from build123d import *

# Parameters (mm, degrees)
SKETCH_R    = 4
PAD_DEPTH   = 14
SKETCH001_R = 2.5
HOLE_DEPTH  = 25
HOLE_TIPS_R = 2.5
FILLET_R    = 1


with BuildPart() as part:
    # Sketch → Pad (new body)
    with BuildSketch(Plane.XY):
        Polygon((0, 0), (25, 0), (25, 8), (14, 8), (14, 36), (0, 36), align=None)
        with Locations((7, 28)):
            Circle(SKETCH_R, mode=Mode.SUBTRACT)
    extrude(amount=PAD_DEPTH)

    # Sketch001 (on Face6 of Pad) → Hole (cut)
    with BuildSketch(Plane(origin=(0, 0, 0), x_dir=(0, -1, 0), z_dir=(-1, 0, 0))):
        with Locations((-13, 7)):
            Circle(SKETCH001_R)
    extrude(amount=-HOLE_DEPTH, mode=Mode.SUBTRACT)

    # Hole tips → Hole tip 1 section 0
    with BuildSketch(Plane(origin=(25, 0, 0), x_dir=(0, -1, 0), z_dir=(-1, 0, 0)), mode=Mode.PRIVATE) as hole_tip_1_s0:
        with Locations((-13, 7)):
            Circle(HOLE_TIPS_R)
    loft([hole_tip_1_s0.sketch, Vertex(26.502152, 13, 7)], mode=Mode.SUBTRACT)

    # Fillet
    fillet_edges = [part.edges().sort_by_distance(p)[0] for p in [
        (14, 8, 7),
        (14, 36, 7),
        (0, 36, 7),
        (25, 8, 7),
    ]]
    fillet(fillet_edges, radius=FILLET_R)


solid = part.part
Can you work these out from the model? Positions are in its coordinate system, mm. A direction names the side the tool comes from. Coordinates: 2 decimals unless noted, no trailing zeros. Order: outer loops, then holes, each group sorted by start corner. A loop starts at its lowest first (then second) coordinate and runs counter-clockwise, first axis right, second up. Notation, with made-up numbers: (55, 77) - (95, 77) arc R26 ccw to (95, 103) - close; hole circle Ø6 at (8, 0). An arc over 180 degrees is marked (long way). Answer as a JSON object with one key per item and string values. Group by question number.
Q1. Imagine slicing it at C-C (x = 11.75). Please give me the cut outline in (y, z), and give its area (3 significant figures).
Q2. Imagine slicing it at A-A (z = 7). Please give me the cut outline in (x, y), and give its area (3 significant figures).
Q3. On a 3-axis mill with a long thin cutter (end or side, diameter ignored), from which of +Z, -Z, +X, -X, +Y, -Y can I reach the whole of each face in a straight line? I mean faces 1 (the face through (0, 18, 7)), 2 (the face through (14, 22, 7)). Say none if no direction works.
Q4. Imagine slicing it at B-B (y = 13). Please give me the cut outline in (x, z).
Q5. I need wall thicknesses on line 1 (Y direction, x = 12, z = 8.5); line 2 (Y direction, x = 4.75, z = 5); line 3 (Z direction, x = 5, y = 13). Which ranges of each line are inside material? Lowest first, please. Write a range as from..to.
Q6. Will these pins go through, and if not, where does the flat tip stop? P1, Ø7, axis at x = 20, z = 4.5, coming from the +Y side; P2, Ø1, axis at y = 21, z = 11, coming from the +X side.
Q7. We'd pull the mould along Z, two halves only. Please class faces 3 (the face through (10, 14, 14)), 4 (the face through (20, 8, 7)), 5 (the face through (6.9, 15, 5.5)): +Z half, -Z half, draft (parallel to the pull), parting line (faces both ways), or undercut.
Q8. Imagine slicing it at D-D (z = 5). Please give me the cut outline in (x, y).
Determined:
{
 "1": {"outline": "(0, 0) - (36, 0) - (36, 14) - (0, 14) - close; hole circle Ø5 at (13, 7)", "area": "484 mm2"},
 "2": {"outline": "(0, 0) - (25, 0) - (25, 7) arc R1 ccw to (24, 8) - (15, 8) arc R1 cw to (14, 9) - (14, 10.5) - (0, 10.5) - close; (0, 15.5) - (14, 15.5) - (14, 35) arc R1 ccw to (13, 36) - (1, 36) arc R1 ccw to (0, 35) - close; hole circle Ø8 at (7, 28)", "area": "471 mm2"},
 "3": {"face 1": "+Z, -Z, -X, +Y, -Y", "face 2": "+Z, -Z, +X, +Y"},
 "4": {"outline": "(0, 0) - (14, 0) - (14, 4.5) - (0, 4.5) - close; (0, 9.5) - (14, 9.5) - (14, 14) - (0, 14) - close"},
 "5": {"line 1": "y = 0..11, 15..36", "line 2": "y = 0..11.5, 14.5..24.69, 31.31..36", "line 3": "z = 0..4.5, 9.5..14"},
 "6": {"P1": "stops at y = 8", "P2": "stops at x = 14"},
 "7": {"face 3": "+Z half", "face 4": "draft", "face 5": "undercut"},
 "8": {"outline": "(0, 0) - (25, 0) - (25, 7) arc R1 ccw to (24, 8) - (15, 8) arc R1 cw to (14, 9) - (14, 11.5) - (0, 11.5) - close; (0, 14.5) - (14, 14.5) - (14, 35) arc R1 ccw to (13, 36) - (1, 36) arc R1 ccw to (0, 35) - close; hole circle Ø8 at (7, 28)"}
}
